Part print with two shaded views. Sizes in mm from the minimum x, y, z corner. A direction names the side the tool comes from. Give positions to 0.01 mm unless a question says otherwise; leave off trailing zeros. Loops run counter-clockwise (first coordinate to the right, second up) from the corner with the lowest first, then second, coordinate; pieces in that order, holes last. Notation, with made-up numbers: (-31.75, 49) -> (18.25, 49) arc R36 ccw to (18.25, 85) -> close; hole circle Ø7 at (-24.75, -2.75). An arc over 180 degrees is marked (long way). One line per question, with ' | ' between items. Start each with the question number.
(1) Mould opens along Z. For the marked faces 1, 2, 3 and 4 say: pulls with the +Z half, pulls with the -Z half, needs draft (parallel to the pull), parting line crosses it, or undercut.
(2) Slice it at C-C, the plane z = 3.75. Write the cut outline in (x, y).
(3) Flat gauge pins, fed straight in: pin 1 Ø1 at (y, z) = (3, 4) entering from +X; pin 2 Ø1.5 at (x, y) = (3.5, 1.5) entering from -Z; pin 3 Ø2.5 at (x, z) = (7, 7.5) entering from +Y. Where does each tip first touch, or does it go through?
(4) Slice it at B-B, the plane x = 6. Write the cut outline in (y, z), then the cut area to 3 significant figures.
(5) 3-axis set-ups, long thin cutter, end or side, ignore diameter. For the marked faces 5 and 6: which of +Z, -Z, +X, -X, +Y, -Y reach the whole face in a straight line?
(6) Drill centre lines: L1, parallel to Z at x = 8.5, y = 3.5; L2, parallel to X at y = 3, z = 4.75. Where is each one in solid material? Low to high. Write a range as from..to.
(7) Slice it at A-A, the plane y = 2. Write the cut outline in (x, z).
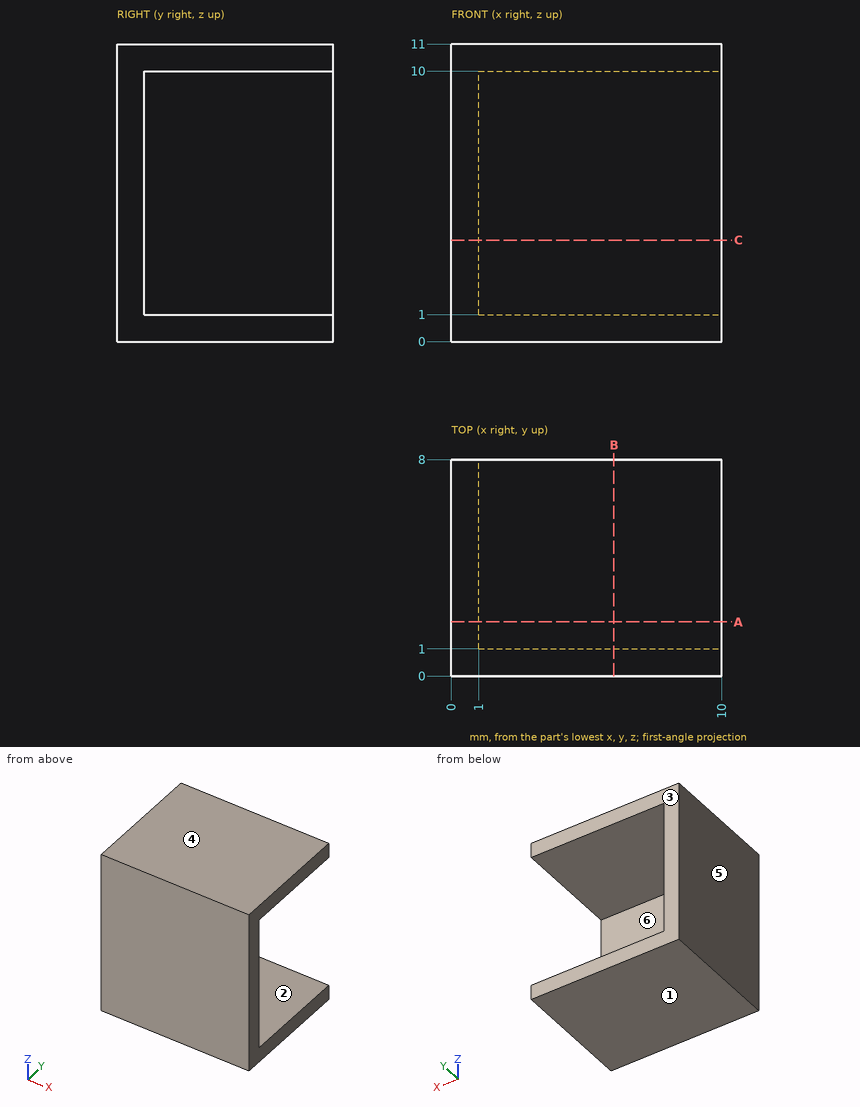
Final values:
1) face 1: pulls with the -Z half | face 2: undercut | face 3: needs draft | face 4: pulls with the +Z half
2) outline: (0, 0) -> (10, 0) -> (10, 1) -> (1, 1) -> (1, 8) -> (0, 8) -> close
3) pin 1: x = 1 | pin 2: z = 0 | pin 3: y = 1
4) outline: (0, 0) -> (8, 0) -> (8, 1) -> (1, 1) -> (1, 10) -> (8, 10) -> (8, 11) -> (0, 11) -> close | area: 25.0 mm2
5) face 5: +Z, -Z, -X, +Y, -Y | face 6: +X, +Y
6) L1: 0..1, 10..11 | L2: 0..1
7) outline: (0, 0) -> (10, 0) -> (10, 1) -> (1, 1) -> (1, 10) -> (10, 10) -> (10, 11) -> (0, 11) -> close
